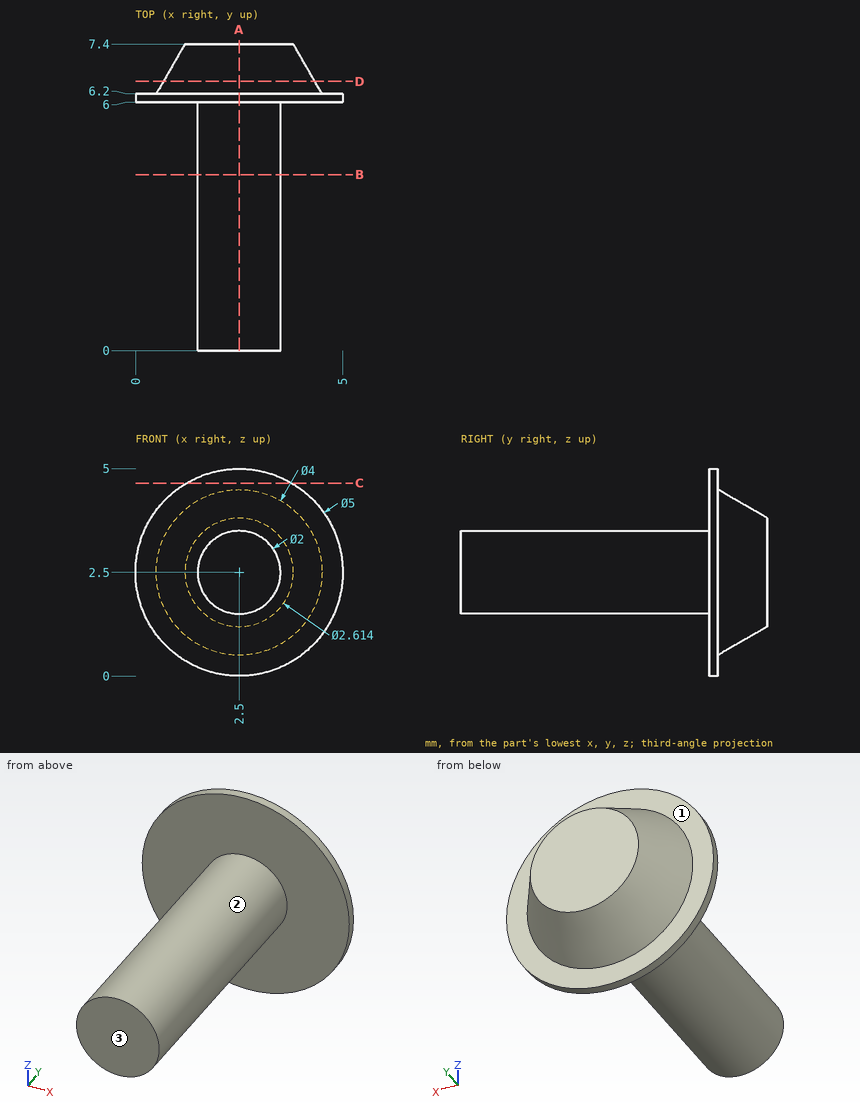
Answer from the drawing. Dimensions are ordinates in mm from the lowest x, y and z of the part. A direction names the side the tool comes from. Round coordinates to 2 decimals unless told otherwise and drop trailing zeros. Loops run counter-clockwise (first coordinate to the right, second up) from the corner with the lowest first, then second, coordinate; pieces in that order, holes last. Notation, with made-up numbers: (89.5, -28) - (147.5, -28) arc R32 cw to (147.5, 3) - close; hole circle Ø1 at (-13, 58.5). An arc over 180 degrees is marked (long way). One line per item, written item: value.
Q1. Find section C-C on z = 4.65. Give the vertices of the cut face in (x, y).
Check values:
outline: (1.22, 6) - (3.78, 6) - (3.78, 6.2) - (1.22, 6.2) - close
Q2. Straight lines are drawn through the part: probe 1 along Y at (x, z) = (3.6, 0.55); probe 2 along Y at (x, z) = (3.7, 2.15); probe 3 along Z at (x, y) = (3.45, 7). For each, find the intervals that lie inside material, in ascending order.
Check values:
probe 1: 6 to 6.2
probe 2: 6 to 7.4
probe 3: 1.29 to 3.71
Q3. Each of these flat-tipped pins is pushed along its axis until it touches: pin 1 Ø1 at (y, z) = (3.5, 2) entering from -X; pin 2 Ø1.5 at (x, z) = (0.5, 4.5) entering from -Y; pin 3 Ø1.5 at (y, z) = (1, 3) entering from +X. Where does it stop, or does it pass through?
Check values:
pin 1: x = 1.5
pin 2: y = 6
pin 3: x = 3.5
Q4. For the marked faces 1, 2 and 3, determine the directions among +Z, -Z, +X, -X, +Y, -Y from which every point of the face is accessible in a straight line to the end or side of a thin tool.
Check values:
face 1: +Y
face 2: -Y
face 3: +Z, -Z, +X, -X, -Y
Q5. Find section A-A on x = 2.5. Give the vertices of the cut face in (y, z), and give its area (3 significant figures).
Check values:
outline: (0, 1.5) - (6, 1.5) - (6, 0) - (6.2, 0) - (6.2, 0.5) - (7.4, 1.19) - (7.4, 3.81) - (6.2, 4.5) - (6.2, 5) - (6, 5) - (6, 3.5) - (0, 3.5) - close
area: 17.0 mm2
Q6. Find section B-B on y = 4.25. Give the vertices of the cut face in (x, z).
Check values:
outline: circle Ø2 at (2.5, 2.5)
Q7. Find section D-D on y = 6.5. Give the vertices of the cut face in (x, z).
Check values:
outline: circle Ø3.65 at (2.5, 2.5)
